Source: CAD feature listing. Evaluate the final solid. Frame: model axes, mm. A direction names the side the tool comes from. Give positions to 0.01 mm unless a question says otherwise; leave off trailing zeros. Write each loop counter-clockwise with the first axis right and the second up, starting at its lowest first coordinate (ties: lowest second). Pieces come first, ordered by that corner, then holes. Notation, with made-up numbers: (1.5, -22) -> (19.5, -22) arc R16 cw to (19.5, -18) -> close; hole circle Ø9 at (73.5, 36.5). An arc over 180 degrees is marked (long way). Answer as a JSON object with one key per item and string values. Group by question number.
Item 1: Ray query, probe 1 along Z at (x, y) = (0, -9.5) (3 decimals); probe 2 along X at (y, z) = (-9.25, -4); probe 3 along Z at (x, y) = (-7, -9.5). Return the intervals inside material, ascending. Write a range as from..to.
Item 2: Pull-direction query (X, two-part tool) for faces 4 (the face through (-11.012, -9.392, -49.592)), 5 (the face through (-1.38, -3.22, -6.2)), 6 (the face through (-2, 0, 3)); classes: pulls with the +X half, pulls with the -X half, needs draft (parallel to the pull), parting line crosses it, or undercut.
Item 3: Section query A-A on z = 0. Give the number of separate pieces and of enclosed holes in the cut face, plus the area to 3 significant figures.
Item 4: Access query for faces 1 (the face through (36.534, -3.131, -28.013)), 2 (the face through (-36.534, -15.919, -28.013)), 3 (the face through (-1.24, -9.57, 44.37)). Directions: +Z, -Z, +X, -X, +Y, -Y. A direction counts if a zero-diameter tool reaches every point of the face in a straight line with its end or side. Return the directions, or none.
Item 5: Section query C-C on x = 23. Return the cut outline in (y, z), plus the area to 3 significant figures.
Item 6: First-contact query: pin 1 Ø8 at (x, z) = (8.5, -17) entering from -Y; pin 2 Ø2 at (y, z) = (-12, 14.5) entering from -X; pin 3 Ø2 at (x, z) = (10.5, -2) entering from +Y; pin 4 Ø11.5 at (x, z) = (24.7, 24.7) entering from -Y. Flat tips, straight axial feed; report the tip coordinate or a pass-through.
from build123d import *

# Parameters (mm, degrees)
F0_R           = 50.8
F1_DEPTH       = 19.05
F2_R           = 3.175
F3_DEPTH       = 19.051
F4_R           = 9.525
F5_DEPTH       = 19.051
F6_R           = 46.0375
F6_R_2         = 9.525
F6_R_3         = 3.175
F7_DEPTH       = 6.35
F8_R           = 46.0375
F8_R_2         = 9.525
F8_R_3         = 3.175
F9_DEPTH       = 6.35
F10_R          = 6.35
F10_R_2        = 3.175
F11_DEPTH      = 6.35
F11_DEPTH_BACK = 12.7


with BuildPart() as f1:
    # F0 (on Front) → F1 (new body)
    with BuildSketch(Plane.XZ):
        Circle(F0_R)
    extrude(amount=F1_DEPTH)

    # F2 (on face) → F3 (cut, through all)
    with BuildSketch(Plane.XZ.offset(19.05)):
        Circle(F2_R)
    extrude(amount=-F3_DEPTH, mode=Mode.SUBTRACT)

    # F4 (on face) → F5 (cut, through all)
    with BuildSketch(Plane.XZ.offset(19.05)):
        with Locations((-24.6957043329, 24.6957043329)):
            Circle(F4_R)
        with Locations((0, 34.925)):
            Circle(F4_R)
        with Locations((24.6957043329, -24.6957043329)):
            Circle(F4_R)
        with Locations((0, -34.925)):
            Circle(F4_R)
        with Locations((-24.6957043329, -24.6957043329)):
            Circle(F4_R)
        with Locations((-34.925, 0)):
            Circle(F4_R)
        with Locations((24.6957043329, 24.6957043329)):
            Circle(F4_R)
        with Locations((34.925, 0)):
            Circle(F4_R)
    extrude(amount=-F5_DEPTH, mode=Mode.SUBTRACT)

    # F6 (on face) → F7 (cut)
    with BuildSketch(Plane.XZ.offset(19.05)):
        Circle(F6_R)
        with Locations((0, -34.925)):
            Circle(F6_R_2, mode=Mode.SUBTRACT)
        with Locations((-34.925, 0)):
            Circle(F6_R_2, mode=Mode.SUBTRACT)
        with Locations((-24.6957043329, -24.6957043329)):
            Circle(F6_R_2, mode=Mode.SUBTRACT)
        Circle(F6_R_3, mode=Mode.SUBTRACT)
        with Locations((24.6957043329, -24.6957043329)):
            Circle(F6_R_2, mode=Mode.SUBTRACT)
        with Locations((34.925, 0)):
            Circle(F6_R_2, mode=Mode.SUBTRACT)
        with Locations((-24.6957043329, 24.6957043329)):
            Circle(F6_R_2, mode=Mode.SUBTRACT)
        with Locations((0, 34.925)):
            Circle(F6_R_2, mode=Mode.SUBTRACT)
        with Locations((24.6957043329, 24.6957043329)):
            Circle(F6_R_2, mode=Mode.SUBTRACT)
    extrude(amount=-F7_DEPTH, mode=Mode.SUBTRACT)

    # F8 (on face) → F9 (cut)
    with BuildSketch(Plane(origin=(0, 0, 0), x_dir=(-1, 0, 0), z_dir=(0, 1, 0))):
        Circle(F8_R)
        with Locations((0, -34.925)):
            Circle(F8_R_2, mode=Mode.SUBTRACT)
        with Locations((-34.925, 0)):
            Circle(F8_R_2, mode=Mode.SUBTRACT)
        with Locations((-24.6957043329, -24.6957043329)):
            Circle(F8_R_2, mode=Mode.SUBTRACT)
        Circle(F8_R_3, mode=Mode.SUBTRACT)
        with Locations((24.6957043329, -24.6957043329)):
            Circle(F8_R_2, mode=Mode.SUBTRACT)
        with Locations((34.925, 0)):
            Circle(F8_R_2, mode=Mode.SUBTRACT)
        with Locations((-24.6957043329, 24.6957043329)):
            Circle(F8_R_2, mode=Mode.SUBTRACT)
        with Locations((0, 34.925)):
            Circle(F8_R_2, mode=Mode.SUBTRACT)
        with Locations((24.6957043329, 24.6957043329)):
            Circle(F8_R_2, mode=Mode.SUBTRACT)
    extrude(amount=-F9_DEPTH, mode=Mode.SUBTRACT)

    # F10 (on face) → F11 (join, two sides)
    with BuildSketch(Plane.XZ.offset(12.7)) as f11_sk:
        Circle(F10_R)
        Circle(F10_R_2, mode=Mode.SUBTRACT)
    extrude(amount=F11_DEPTH)
    extrude(f11_sk.sketch, amount=-F11_DEPTH_BACK)


solid = f1.part
Worked answers:
{
 "1": {"probe 1": "-50.8..-44.45, -25.4..-3.175, 3.175..25.4, 44.45..50.8", "probe 2": "-50.64..-43.57, -26.28..26.28, 43.57..50.64", "probe 3": "-50.32..-41.38, -28.47..28.47, 41.38..50.32"},
 "2": {"face 4": "parting line crosses it", "face 5": "undercut", "face 6": "needs draft"},
 "3": {"separate pieces": "4", "enclosed holes": "0", "area": "565 mm^2"},
 "4": {"face 1": "+Y", "face 2": "-Y", "face 3": "+Y, -Y"},
 "5": {"outline": "(-19.05, -45.3) -> (0, -45.3) -> (0, -39.88) -> (-6.35, -39.88) -> (-6.35, -34.07) -> (-12.7, -34.07) -> (-12.7, -39.88) -> (-19.05, -39.88) -> close; (-19.05, 39.88) -> (-12.7, 39.88) -> (-12.7, 34.07) -> (-6.35, 34.07) -> (-6.35, 39.88) -> (0, 39.88) -> (0, 45.3) -> (-19.05, 45.3) -> close; (-12.7, -15.32) -> (-6.35, -15.32) -> (-6.35, 15.32) -> (-12.7, 15.32) -> close", "area": "475 mm^2"},
 "6": {"pin 1": "y = -12.7", "pin 2": "x = -48.97", "pin 3": "y = -6.35", "pin 4": "through"}
}
